from build123d import *

# Parameters (mm, degrees)
BOSS_EXTRUDE1_DEPTH = 6


with BuildPart() as part:
    # Sketch1 → Boss-Extrude1 (new body)
    with BuildSketch(Plane(origin=(0, 0, 0), x_dir=(1, 0, 0), z_dir=(0, 1, 0))):
        with BuildLine():
            Line((-43.714285714, -124.928571429), (-43.714285714, -118.928571429))
            Line((-43.714285714, -118.928571429), (-67.714285714, -118.928571429))
            Line((-67.714285714, -118.928571429), (-67.714285714, -124.928571429))
            Line((-67.714285714, -124.928571429), (-91.714285714, -124.928571429))
            Line((-91.714285714, -124.928571429), (-91.714285714, -118.928571429))
            Line((-91.714285714, -118.928571429), (-104.714285714, -118.928571429))
            Line((-104.714285714, -118.928571429), (-104.714285714, -76.928571429))
            Line((-104.714285714, -76.928571429), (-110.714285714, -76.928571429))
            Line((-110.714285714, -76.928571429), (-110.714285714, -34.928571429))
            Line((-110.714285714, -34.928571429), (-104.714285714, -34.928571429))
            Line((-104.714285714, -34.928571429), (-104.714285714, 7.071428571))
            Line((-104.714285714, 7.071428571), (-110.714285714, 7.071428571))
            Line((-110.714285714, 7.071428571), (-110.714285714, 49.071428571))
            Line((-110.714285714, 49.071428571), (-104.714285714, 49.071428571))
            Line((-104.714285714, 49.071428571), (-104.714285714, 79.071428571))
            Line((-104.714285714, 79.071428571), (-79.714285714, 79.071428571))
            Line((-79.714285714, 79.071428571), (-79.714285714, 85.071428571))
            Line((-79.714285714, 85.071428571), (-104.714285714, 85.071428571))
            Line((-104.714285714, 85.071428571), (-104.714285714, 91.071428571))
            Line((-104.714285714, 91.071428571), (83.285714286, 91.071428571))
            Line((83.285714286, 91.071428571), (83.285714286, 85.071428571))
            Line((83.285714286, 85.071428571), (58.285714286, 85.071428571))
            Line((58.285714286, 85.071428571), (58.285714286, 79.071428571))
            Line((58.285714286, 79.071428571), (83.285714286, 79.071428571))
            Line((83.285714286, 79.071428571), (83.285714286, 49.071428571))
            Line((83.285714286, 49.071428571), (89.285714286, 49.071428571))
            Line((89.285714286, 49.071428571), (89.285714286, 7.071428571))
            Line((89.285714286, 7.071428571), (83.285714286, 7.071428571))
            Line((83.285714286, 7.071428571), (83.285714286, -34.928571429))
            Line((83.285714286, -34.928571429), (89.285714286, -34.928571429))
            Line((89.285714286, -34.928571429), (89.285714286, -76.928571429))
            Line((89.285714286, -76.928571429), (83.285714286, -76.928571429))
            Line((83.285714286, -76.928571429), (83.285714286, -79.166780724))
            ThreePointArc((83.285714286, -79.166780724), (23.663965975, -68.356840195), (-9.714285714, -118.928571429))
            Line((-9.714285714, -118.928571429), (-19.714285714, -118.928571429))
            Line((-19.714285714, -118.928571429), (-19.714285714, -124.928571429))
            Line((-19.714285714, -124.928571429), (-43.714285714, -124.928571429))
        make_face()
    extrude(amount=BOSS_EXTRUDE1_DEPTH)


solid = part.part
The listing builds one solid part. Answer for the finished solid, in the listing's coordinates (mm). A direction names the side the tool comes from. Round coordinates to 2 decimals unless told otherwise and drop trailing zeros. Order: outer loops, then holes, each group sorted by start corner. A loop starts at its lowest first (then second) coordinate and runs counter-clockwise, first axis right, second up. Notation, with made-up numbers: (72, -34.75) - (121, -34.75) arc R19 ccw to (121, -14.75) - close; hole circle Ø9 at (74, 67). An arc over 180 degrees is marked (long way). Write item = value, one per line. Start each with the question number.
1) Straight lines are drawn through the part: L1, parallel to Z at x = -101, y = 5.6; L2, parallel to X at y = 2.25, z = -7; L3, parallel to Z at x = -17, y = 4.6. For each, find the intervals that lie inside material, in ascending order.
2) Section B-B, the plane z = 30.5 is taken. Write down the section's boundary in (x, y).
3) For a pull along Z with two mould halves and no side action, classify faces 4 (the flat face through (-9, 0, 15)), 5 (the flat face through (86, 3, 34.929)), 6 (the flat face through (86, 3, -49.071)), 7 (the cylindrical face through (24.49, 2.96, 68.01)) as released by +Z, released by -Z, zero draft, split by the parting line, or undercut.
4) Section A-A, the plane x = -82.5 is taken. Write down the section's boundary in (y, z).
5) Given pin 1 (1.8 mm diameter, centred on y = 4.5, z = 121, fed in from -X); pin 2 (1.8 mm diameter, centred on y = 2, z = -83, fed in from -X); pin 3 (1.8 mm diameter, centred on y = 3.5, z = -65, fed in from -X); pin 4 (3 mm diameter, centred on x = -52, z = 61.5, fed in from -Y), each flat-ended and moving along its own axis, determine where each tip first touches the part or whether it passes through.
6) Section C-C, the plane x = -48 is taken. Write down the section's boundary in (y, z).
7) For faces 1 (the flat face through (83.286, 3, 14)), 2 (the flat face through (-104.714, 3, 14)), 3 (the flat face through (-56, 3, 118.929)), determine the directions among +Z, -Z, +X, -X, +Y, -Y from which every point of the face is accessible in a straight line to the end or side of a thin tool.
Results list:
q1.L1 = -91.07 to -85.07, -79.07 to 118.93
q1.L2 = -104.71 to 83.29
q1.L3 = -91.07 to 118.93
q2.outline = (-104.71, 0) - (83.29, 0) - (83.29, 6) - (-104.71, 6) - close
q3.face_4 = zero draft
q3.face_5 = undercut
q3.face_6 = released by -Z
q3.face_7 = released by +Z
q4.outline = (0, -91.07) - (6, -91.07) - (6, -85.07) - (0, -85.07) - close; (0, -79.07) - (6, -79.07) - (6, 124.93) - (0, 124.93) - close
q5.pin_1 = -91.71
q5.pin_2 = -79.71
q5.pin_3 = -104.71
q5.pin_4 = 0
q6.outline = (0, -91.07) - (6, -91.07) - (6, 118.93) - (0, 118.93) - close
q7.face_1 = +X, +Y, -Y
q7.face_2 = -X, +Y, -Y
q7.face_3 = +Z, +Y, -Y
